For this review, take the finished solid that the model builds, in its own axes (mm). A direction names the side the tool comes from. Give positions to 0.01 mm unless a question says otherwise; leave off trailing zeros. Loops run counter-clockwise (first coordinate to the right, second up) from the corner with the lowest first, then second, coordinate; pieces in that order, holes last. Notation, with made-up numbers: M -15.5,61 L 10.5,61 A16 cw 10.5,72 Z; hole C -23,-7 d2. An arc over 180 degrees is marked long. Use CSV: the item, a comma, the result in double quotes. Start each with the question number.
1. Insertion check: P1, Ø6, axis at x = -13.5, z = -9, coming from the +Y side; P2, Ø10, axis at x = -57, z = -3, coming from the +Y side; P3, Ø2, axis at x = 0.5, z = -13, coming from the +Y side. Each pin has a flat end and moves straight along its axis. Give the tip position at first contact, or say it passes through.
2. The part is to be moulded in two halves that separate along Z. For faces 1 (the face through (-33, 7, -32)), 2 (the face through (-33, 15, 2)), 3 (the face through (1, 5, -15)), 4 (the face through (2, 8, 2)), say which applies: pulls with the +Z half, pulls with the -Z half, needs draft (parallel to the pull), parting line crosses it, or undercut.
3. Tool access review of faces 5 (the face through (-66, 5, -15)), 6 (the face through (-32, 4, -14)), 7 (the face through (2, 7, -31)): name each direction out of +Z, -Z, +X, -X, +Y, -Y from which nothing blocks a thin tool from reaching the whole face with its end or side.
4. Take a section at B-B, the plane y = 6.5. Write out the cut boundary in (x, z), and give its area (3 significant figures).
5. To check wall thickness, follow line 1 (Z direction, x = -27.5, y = 8.25); line 2 (X direction, y = 4.75, z = -8); line 3 (Y direction, x = -8.5, z = -12). State the ranges of each line that lie inside material, in increasing order. Write a range as [from, to].
6. Take a section at C-C, the plane z = -2.5. Write out the cut boundary in (x, y), and give its area (3 significant figures).
7. Take a section at A-A, the plane x = -14.5. Write out the cut boundary in (y, z), and give its area (3 significant figures).
Autodesk Inventor part; units mm, degrees
ref_plane "YZ Plane" through (0, 0, 0) normal (1, 0, 0) x (0, 1, 0)
ref_plane "XZ Plane" through (0, 0, 0) normal (0, 1, 0) x (-1, 0, 0)
ref_plane "XY Plane" through (0, 0, 0) normal (0, 0, 1) x (1, 0, 0)
sketch "Sketch1" plane through (0, 0, 0) normal (0, 1, 0) x (-1, 0, 0)
  line L0 (0, 0) -> (0, -29)
  line L1 (0, 0) -> (65, 0)
  line L2 (65, 0) -> (65, -29)
  line L3 (65, -29) -> (0, -29)
  dimension "d0" = 29
  dimension "d1" = 65
extrude "Extrusion1" add sketch "Sketch1" along normal blind 4
sketch "Sketch3" plane through (0, 0, 0) normal (0, -1, 0) x (1, 0, 0)
  line L0 (0, 0) -> (0, -29)
  line L1 (-65, 0) -> (0, 0)
  line L2 (-65, -29) -> (-65, 0)
  line L3 (0, -29) -> (-65, -29)
  line L4 (3, -32) -> (3, 3)
  line L5 (3, 3) -> (-68, 3)
  line L6 (-68, 3) -> (-68, -32)
  line L7 (-68, -32) -> (3, -32)
  dimension "d4" = 3
extrude "Extrusion2" add sketch "Sketch3" against normal blind 15
sketch "Sketch4" plane through (3, 0, 3) normal (1, 0, 0) x (0, 0, -1)
  line L0 (3, 4) -> (32, 4)
  line L1 (32, 4) -> (3, 4)
  line L2 (3, 4) -> (3, 15)
  line L3 (32, 4) -> (32, 15)
  line L4 (3, 4) -> (32, 4)
  line L5 (3, 15) -> (32, 15)
  line L6 (0, 15) -> (35, 15)
  point P0 (3, 0)
extrude "Extrusion3" cut sketch "Sketch4" against normal blind 72.15
chamfer "Chamfer1" distance 2 angle 45 4 edges at (3, 7.5, 3) (-68, 7.5, 3) (-68, 7.5, -32) (3, 7.5, -32)
sketch "Sketch5" plane through (0, 4, 0) normal (0, 1, 0) x (1, 0, 0)
  line L0 (-68, 0) -> (-68, 29)
  line L1 (3, 29) -> (3, 0)
  line L2 (-68, 29) -> (3, 29)
  line L3 (-1, 29) -> (-1, 0)
  line L4 (-64, 29) -> (-64, 0)
  line L5 (3, 0) -> (-68, 0)
  point P0 (0, 0)
extrude "Extrusion4" add sketch "Sketch5" along normal blind 1 contours L0 L2 L4 L5 | L3 L2 L1 L5
properties part number "Buck Converter Holder"
Result set:
1,P1,"y = 4"
1,P2,"y = 15"
1,P3,"y = 5"
2,face 1,"pulls with the -Z half"
2,face 2,"needs draft"
2,face 3,"undercut"
2,face 4,"pulls with the +Z half"
3,face 5,"+X, -X, +Y"
3,face 6,"+Y"
3,face 7,"-Z, +X, +Y, -Y"
4,outline,"M -68,-30 L -66,-32 L 1,-32 L 3,-30 L 3,-29 L -68,-29 Z; M -68,0 L 3,0 L 3,1 L 1,3 L -66,3 L -68,1 Z"
4,area,"418 mm2"
5,line 1,"[-32, -29], [0, 3]"
5,line 2,"[-68, -64], [-1, 3]"
5,line 3,"[0, 4]"
6,outline,"M -68,0 L 3,0 L 3,5 L -1,5 L -1,4 L -64,4 L -64,5 L -68,5 Z"
6,area,"292 mm2"
7,outline,"M 0,-32 L 15,-32 L 15,-29 L 4,-29 L 4,0 L 15,0 L 15,3 L 0,3 Z"
7,area,"206 mm2"
